```python
from build123d import *

# Parameters (mm, degrees)
BASE_DEPTH  = 96
ESQUISSE2_R = 2.5
TROU_DEPTH  = 98.037363938


with BuildPart() as part:
    # Esquisse1 → BASE (new body)
    with BuildSketch(Plane(origin=(0, 0, 0), x_dir=(1, 0, 0), z_dir=(0, 1, 0))):
        Polygon((-2, -3.75), (-2, 2.75), (2, 2.75), (2, -3.75), (12, -3.75), (12, 3.75), (-12, 3.75), (-12, -3.75), align=None)
    extrude(amount=-BASE_DEPTH)

    # Esquisse2 → TROU (cut, through all)
    with BuildSketch(Plane.XY.offset(3.75)):
        with Locations((-7, -8)):
            Circle(ESQUISSE2_R)
        with Locations((7, -8)):
            Circle(ESQUISSE2_R)
        with Locations((7, -24)):
            Circle(ESQUISSE2_R)
        with Locations((7, -40)):
            Circle(ESQUISSE2_R)
        with Locations((7, -56)):
            Circle(ESQUISSE2_R)
        with Locations((7, -72)):
            Circle(ESQUISSE2_R)
        with Locations((7, -88)):
            Circle(ESQUISSE2_R)
        with Locations((-7, -24)):
            Circle(ESQUISSE2_R)
        with Locations((-7, -40)):
            Circle(ESQUISSE2_R)
        with Locations((-7, -56)):
            Circle(ESQUISSE2_R)
        with Locations((-7, -72)):
            Circle(ESQUISSE2_R)
        with Locations((-7, -88)):
            Circle(ESQUISSE2_R)
    extrude(amount=-TROU_DEPTH, mode=Mode.SUBTRACT)


solid = part.part
```
Source: CAD feature listing. Evaluate the final solid. Frame: model axes, mm. A direction names the side the tool comes from. Coordinates: 2 decimals unless noted, no trailing zeros. Loops run counter-clockwise (first coordinate to the right, second up) from the corner with the lowest first, then second, coordinate; pieces in that order, holes last. Notation, with made-up numbers: (-9, -17.75) -> (37, -17.75) arc R30 cw to (37, 19.25) -> close; hole circle Ø8 at (36, 37). An arc over 180 degrees is marked (long way). One line per item, written item: value. Start each with the question number.
Q1. Section query C-C, the plane z = -0.25. Give the number of separate pieces and of enclosed holes in the cut face, and give its area (3 significant figures).
Q2. Section query B-B, the plane y = -38.5. Return the cut outline in (x, z), and give its area (3 significant figures).
Q3. Mould query, pull axis Y, two halves, no side actions, for faces 1 (the face through (-7, -47, 3.75)), 2 (the face through (2.5, -96, -0.1)), 3 (the face through (-5.66, -21.89, 0.05)). Classes: pulls with the +Y half, pulls with the -Y half, needs draft (parallel to the pull), parting line crosses it, or undercut.
Q4. Section query D-D, the plane y = -81. Return the cut outline in (x, z), and give its area (3 significant figures).
Q5. Set-up query: faces 4 (the face through (-2, -47, 1)), 5 (the face through (8.15, -10.22, 0.05)). Return all of +Z, -Z, +X, -X, +Y, -Y with unobstructed straight access to the full face (end or side cutting, diameter ignored); none if empty.
Q6. Line query: line 1 along X through (y, z) = (-19, 2.25); line 2 along X through (y, z) = (-70, 2.75). Output: solid intervals per line, ascending.
Q7. Section query A-A, the plane x = 7. Return the cut outline in (y, z), and give its area (3 significant figures).
Results:
1. separate pieces: 2
1. enclosed holes: 12
1. area: 1,680 mm^2
2. outline: (-12, -3.75) -> (-9, -3.75) -> (-9, 3.75) -> (-12, 3.75) -> close; (-5, -3.75) -> (5, -3.75) -> (5, 3.75) -> (2, 3.75) -> (2, -2.75) -> (-2, -2.75) -> (-2, 3.75) -> (-5, 3.75) -> close; (9, -3.75) -> (12, -3.75) -> (12, 3.75) -> (9, 3.75) -> close
2. area: 94.0 mm^2
3. face 1: needs draft
3. face 2: pulls with the -Y half
3. face 3: undercut
4. outline: (-12, -3.75) -> (12, -3.75) -> (12, 3.75) -> (2, 3.75) -> (2, -2.75) -> (-2, -2.75) -> (-2, 3.75) -> (-12, 3.75) -> close
4. area: 154 mm^2
5. face 4: +Z, +Y, -Y
5. face 5: +Z, -Z
6. line 1: -12 to -2, 2 to 12
6. line 2: -12 to -8.5, -5.5 to -2, 2 to 5.5, 8.5 to 12
7. outline: (-96, -3.75) -> (-90.5, -3.75) -> (-90.5, 3.75) -> (-96, 3.75) -> close; (-85.5, -3.75) -> (-74.5, -3.75) -> (-74.5, 3.75) -> (-85.5, 3.75) -> close; (-69.5, -3.75) -> (-58.5, -3.75) -> (-58.5, 3.75) -> (-69.5, 3.75) -> close; (-53.5, -3.75) -> (-42.5, -3.75) -> (-42.5, 3.75) -> (-53.5, 3.75) -> close; (-37.5, -3.75) -> (-26.5, -3.75) -> (-26.5, 3.75) -> (-37.5, 3.75) -> close; (-21.5, -3.75) -> (-10.5, -3.75) -> (-10.5, 3.75) -> (-21.5, 3.75) -> close; (-5.5, -3.75) -> (0, -3.75) -> (0, 3.75) -> (-5.5, 3.75) -> close
7. area: 495 mm^2
